Source: CAD feature listing. Evaluate the final solid. Frame: model axes, mm. A direction names the side the tool comes from. Give positions to 0.01 mm unless a question says otherwise; leave off trailing zeros. Loops run counter-clockwise (first coordinate to the right, second up) from the corner with the lowest first, then second, coordinate; pieces in that order, holes last. Notation, with made-up numbers: (29.5, -39.5) -> (63.5, -39.5) arc R18 ccw to (63.5, -16.5) -> close; hole circle Ø2 at (-15, -5.75). An arc over 180 degrees is marked (long way). Answer as a JSON object with one key per item and string values. Group by question number.
from build123d import *

# Parameters (mm, degrees)
EXTRUDE_THIN1_DEPTH    = 16.002
CUT_EXTRUDE1_START     = -15.748
CUT_EXTRUDE1_OUTLINE_R = 1.3
CUT_EXTRUDE1_DEPTH     = 15.748
BOSS_EXTRUDE2_DEPTH    = 1.68
BOSS_EXTRUDE3_START    = 1.68
BOSS_EXTRUDE3_DEPTH    = 1.68
CUT_EXTRUDE2_START     = -2.384
CUT_EXTRUDE2_DEPTH     = 2.384
CUT_EXTRUDE3_DEPTH     = 2.384
CHAMFER1_SIZE          = 1.7
CHAMFER2_SIZE          = 2.38
SKETCH10_W             = 17
SKETCH10_H             = 13.5
BOSS_EXTRUDE4_DEPTH    = 12
SKETCH11_R             = 5.6
SKETCH11_R_2           = 5
BOSS_EXTRUDE5_DEPTH    = 15
FILLET1_R              = 4


# Read off the part's stored shape, not the designer's step: Cut-Extrude1
with BuildPart() as part:
    # Sketch1 → Extrude-Thin1 (new body)
    with BuildSketch(Plane.XY):
        with BuildLine():
            Line((-42.06875, -12.7), (-35.433, -12.7))
            ThreePointArc((-35.433, -12.7), (-33.636948776, -11.956051224), (-32.893, -10.16))
            Line((-32.893, -10.16), (-32.893, -2.54))
            ThreePointArc((-32.893, -2.54), (-32.149051224, -0.743948776), (-30.353, 0))
            Line((-30.353, 0), (30.353, 0))
            ThreePointArc((30.353, 0), (32.149051224, -0.743948776), (32.893, -2.54))
            Line((32.893, -2.54), (32.893, -10.16))
            ThreePointArc((32.893, -10.16), (33.636948776, -11.956051224), (35.433, -12.7))
            Line((35.433, -12.7), (42.06875, -12.7))
            Line((42.06875, -12.7), (42.06875, -15.748))
            Line((42.06875, -15.748), (35.433, -15.748))
            ThreePointArc((35.433, -15.748), (31.481687307, -14.111312693), (29.845, -10.16))
            Line((29.845, -10.16), (29.845, -3.048))
            Line((29.845, -3.048), (-29.845, -3.048))
            Line((-29.845, -3.048), (-29.845, -10.16))
            ThreePointArc((-29.845, -10.16), (-31.481687307, -14.111312693), (-35.433, -15.748))
            Line((-35.433, -15.748), (-42.06875, -15.748))
            Line((-42.06875, -15.748), (-42.06875, -12.7))
        make_face()
    extrude(amount=-EXTRUDE_THIN1_DEPTH)

    # Cut-Extrude1 outline → Cut-Extrude1 (cut)
    with BuildSketch(Plane(origin=(0, 0, 0), x_dir=(1, 0, 0), z_dir=(0, 1, 0)).offset(CUT_EXTRUDE1_START)):
        with BuildLine():
            Line((35.433, 13.462), (-35.433, 13.462))
            ThreePointArc((-35.433, 13.462), (-37.133, 11.762), (-35.433, 10.062))
            Line((-35.433, 10.062), (-32.893, 10.062))
            Line((-32.893, 10.062), (-32.893, 8.382))
            Line((-32.893, 8.382), (-1.27, 8.382))
            Line((-1.27, 8.382), (-1.27, 12.446))
            Line((-1.27, 12.446), (32.893, 12.446))
            Line((32.893, 12.446), (32.893, 10.062))
            Line((32.893, 10.062), (35.433, 10.062))
            ThreePointArc((35.433, 10.062), (37.133, 11.762), (35.433, 13.462))
        make_face()
        with BuildLine():
            Line((32.893, 5.94), (32.893, 7.62))
            Line((32.893, 7.62), (1.27, 7.62))
            Line((1.27, 7.62), (1.27, 3.556))
            Line((1.27, 3.556), (-32.893, 3.556))
            Line((-32.893, 3.556), (-32.893, 5.94))
            Line((-32.893, 5.94), (-35.433, 5.94))
            ThreePointArc((-35.433, 5.94), (-37.133, 4.24), (-35.433, 2.54))
            Line((-35.433, 2.54), (35.433, 2.54))
            ThreePointArc((35.433, 2.54), (37.133, 4.24), (35.433, 5.94))
            Line((35.433, 5.94), (32.893, 5.94))
        make_face()
        with BuildLine():
            Line((42.06875, 16.002), (35.433, 16.002))
            ThreePointArc((35.433, 16.002), (40.193949205, 13.198335352), (42.06875, 8.001))
            Line((42.06875, 8.001), (42.06875, 16.002))
        make_face()
        with BuildLine():
            Line((42.06875, 0), (42.06875, 8.001))
            ThreePointArc((42.06875, 8.001), (40.193949205, 2.803664648), (35.433, 0))
            Line((35.433, 0), (42.06875, 0))
        make_face()
        with BuildLine():
            ThreePointArc((-42.06875, 8.001), (-40.193949205, 13.198335352), (-35.433, 16.002))
            Line((-35.433, 16.002), (-42.06875, 16.002))
            Line((-42.06875, 16.002), (-42.06875, 8.001))
        make_face()
        with BuildLine():
            ThreePointArc((-35.433, 0), (-40.193949205, 2.803664648), (-42.06875, 8.001))
            Line((-42.06875, 8.001), (-42.06875, 0))
            Line((-42.06875, 0), (-35.433, 0))
        make_face()
        with Locations((38.750875, 8.001)):
            Circle(CUT_EXTRUDE1_OUTLINE_R)
        with Locations((-38.750875, 8.001)):
            Circle(CUT_EXTRUDE1_OUTLINE_R)
    extrude(amount=CUT_EXTRUDE1_DEPTH, mode=Mode.SUBTRACT)

    # Sketch6 → Boss-Extrude2 (add)
    with BuildSketch(Plane(origin=(0, 0, -8.382), x_dir=(-1, 0, 0), z_dir=(0, 0, -1))):
        with BuildLine():
            Line((32.893, -10.16), (32.893, -6.604))
            Line((32.893, -6.604), (29.845, -6.604))
            Line((29.845, -6.604), (29.845, -10.16))
            ThreePointArc((29.845, -10.16), (30.667537588, -13.078237824), (32.893, -15.137363157))
            Line((32.893, -15.137363157), (32.893, -10.16))
        make_face()
    extrude(amount=BOSS_EXTRUDE2_DEPTH)

    # Sketch7 → Boss-Extrude3 (add)
    with BuildSketch(Plane.XY.offset(-7.62).offset(BOSS_EXTRUDE3_START)):
        with BuildLine():
            Line((32.893, -10.16), (32.893, -6.6))
            Line((32.893, -6.6), (29.845, -6.604))
            Line((29.845, -6.604), (29.845, -10.16))
            ThreePointArc((29.845, -10.16), (30.667537588, -13.078237824), (32.893, -15.137363157))
            Line((32.893, -15.137363157), (32.893, -10.16))
        make_face()
    extrude(amount=-BOSS_EXTRUDE3_DEPTH)

    # Sketch8 → Cut-Extrude2 (cut)
    with BuildSketch(Plane(origin=(0, 0, -12.446), x_dir=(-1, 0, 0), z_dir=(0, 0, -1)).offset(CUT_EXTRUDE2_START)):
        with BuildLine():
            Line((-32.893, -15.137363157), (-32.893, -6.6))
            Line((-32.893, -6.6), (-29.845, -6.604))
            Line((-29.845, -6.604), (-29.845, -10.16))
            ThreePointArc((-29.845, -10.16), (-30.667537588, -13.078237824), (-32.893, -15.137363157))
        make_face()
    extrude(amount=CUT_EXTRUDE2_DEPTH, mode=Mode.SUBTRACT)

    # Sketch9 → Cut-Extrude3 (cut)
    with BuildSketch(Plane.XY.offset(-3.556)):
        with BuildLine():
            Line((-32.893, -15.137363157), (-32.893, -6.604))
            Line((-32.893, -6.604), (-29.845, -6.604))
            Line((-29.845, -6.604), (-29.845, -10.16))
            ThreePointArc((-29.845, -10.16), (-30.667537588, -13.078237824), (-32.893, -15.137363157))
        make_face()
    extrude(amount=-CUT_EXTRUDE3_DEPTH, mode=Mode.SUBTRACT)

    # Chamfer1
    # the kernel refuses this chamfer: 1.7 mm, written as the material it adds along each edge
    # the kernel refuses this chamfer: 1.7 mm, written as the material it takes off along each edge
    with BuildSketch(Plane(origin=(-37.26486108, -6.604, -10.062), x_dir=(0, -0.9996219169112968, -0.02749587661058687), z_dir=(1, 0, 0))) as chamfer1_2_piece_1_section:
        Polygon((CHAMFER1_SIZE * 0.999621916911, -CHAMFER1_SIZE * 0.0274958766106), (-CHAMFER1_SIZE * 0.0274958766106, -CHAMFER1_SIZE * 0.999621916911), (0, 0), align=None)
    chamfer1_2_piece_1 = extrude(amount=11.791722159, mode=Mode.PRIVATE)
    chamfer1_2_piece_1 = split(chamfer1_2_piece_1, bisect_by=Plane(origin=(-31.369, -7.170744186, -8.382), z_dir=(0, 0, -1)), keep=Keep.TOP, mode=Mode.PRIVATE)
    add(chamfer1_2_piece_1, mode=Mode.SUBTRACT)
    with BuildSketch(Plane(origin=(37.264857315, -6.594262654, -5.94), x_dir=(0.00131183865632537, -0.9996210561251475, 0.02749587661058631), z_dir=(-0.999999138888279, -0.0013123348279305267, 0))) as chamfer1_2_piece_2_section:
        Polygon((CHAMFER1_SIZE * 0.999621916911, -CHAMFER1_SIZE * 0.0274958766106), (-CHAMFER1_SIZE * 0.0274958766106, -CHAMFER1_SIZE * 0.999621916911), (0, 0), align=None)
    chamfer1_2_piece_2 = extrude(amount=11.791724784, mode=Mode.PRIVATE)
    chamfer1_2_piece_2 = split(chamfer1_2_piece_2, bisect_by=Plane(origin=(31.369, -7.168744674, -7.62), z_dir=(0, 0, 1)), keep=Keep.TOP, mode=Mode.PRIVATE)
    add(chamfer1_2_piece_2, mode=Mode.SUBTRACT)

    # Chamfer2
    chamfer2_edges = [part.edges().sort_by_distance(p)[0] for p in [
        (31.369, -6.602, -10.062),
        (-31.369, -6.604, -5.94),
    ]]
    chamfer(chamfer2_edges, length=CHAMFER2_SIZE)

    # Sketch10 → Boss-Extrude4 (add)
    with BuildSketch(Plane.XZ.offset(3.048)):
        with Locations((-21.345, -8.001)):
            Rectangle(SKETCH10_W, SKETCH10_H)
    extrude(amount=BOSS_EXTRUDE4_DEPTH)

    # Sketch11 → Boss-Extrude5 (add)
    with BuildSketch(Plane(origin=(-12.845, 0, 0), x_dir=(0, 0, -1), z_dir=(1, 0, 0))):
        with Locations(Location((8.001, -9.048, 0), (0, 0, 270))):
            Circle(SKETCH11_R)
        with Locations(Location((8.001, -9.048, 0), (0, 0, 90))):
            Circle(SKETCH11_R_2, mode=Mode.SUBTRACT)
    extrude(amount=BOSS_EXTRUDE5_DEPTH)

    # Fillet1
    fillet1_edges = [part.edges().sort_by_distance(p)[0] for p in [
        (-21.345, -15.048, -14.751),
        (-21.345, -15.048, -1.251),
    ]]
    fillet(fillet1_edges, radius=FILLET1_R)


solid = part.part
(1) Mould query, pull axis Z, two halves, no side actions, for faces 5 (the face through (1.27, -2, -6)), 6 (the face through (32.893, -6, -15)), 7 (the face through (-5.45, -14.221, -5.856)). Classes: pulls with the +Z half, pulls with the -Z half, needs draft (parallel to the pull), parting line crosses it, or undercut.
(2) Section query D-D on x = -19.5. Return the cut outline in (y, z).
(3) Material intervals for line 1 (Z direction, x = -8, y = -2.25); line 2 (X direction, y = -7.75, z = -9.75) (3 decimals); line 3 (Y direction, x = -9, z = -4.25), sorted ascending. Write a range as from..to.
(4) Section query C-C on x = 6. Return the cut outline in (y, z), plus the area to 3 significant figures.
(5) Section query A-A on x = -2.5. Return the cut outline in (y, z), plus the area to 3 significant figures.
(6) First-contact query: pin 1 (8 mm diameter, centred on y = -8, z = -6, fed in from +X); pin 2 (1 mm diameter, centred on x = -32.5, y = -4, fed in from +Z); pin 3 (5 mm diameter, centred on x = 22, z = -2, fed in from -Y); pin 4 (3.5 mm diameter, centred on y = -8, z = -10.5, fed in from +X). Flat tips, straight axial feed; report the tip coordinate or a pass-through.
(7) Access query for faces 1 (the face through (31.525, -14.155, -14.714)), 2 (the face through (32.893, -6, -9)), 3 (the face through (-32.893, -6, -7)), 4 (the face through (0.5, -2.7, -13.462)). Directions: +Z, -Z, +X, -X, +Y, -Y. A direction counts if a zero-diameter tool reaches every point of the face in a straight line with its end or side. Return the directions, or none.
(8) Section query B-B on y = -1.25. Return the cut outline in (x, z).
Result:
{
 "1": {"face 5": "undercut", "face 6": "needs draft", "face 7": "parting line crosses it"},
 "2": {"outline": "(-15.05, -10.75) arc R4 ccw to (-11.05, -14.75) -> (-3.05, -14.75) -> (-3.05, -16) -> (0, -16) -> (0, -13.46) -> (-3.05, -13.46) -> (-3.05, -8.38) -> (0, -8.38) -> (0, -3.56) -> (-3.05, -3.56) -> (-3.05, -2.54) -> (0, -2.54) -> (0, 0) -> (-3.05, 0) -> (-3.05, -1.25) -> (-11.05, -1.25) arc R4 ccw to (-15.05, -5.25) -> close"},
 "3": {"line 1": "-16..-13.46, -8.38..-3.56, -2.54..0", "line 2": "-29.845..-12.845, 29.845..32.893", "line 3": "-13.21..-12.35, -5.74..-4.89, -3.05..0"},
 "4": {"outline": "(-3.05, -16) -> (0, -16) -> (0, -13.46) -> (-3.05, -13.46) -> close; (-3.05, -12.45) -> (0, -12.45) -> (0, -7.62) -> (-3.05, -7.62) -> close; (-3.05, -2.54) -> (0, -2.54) -> (0, 0) -> (-3.05, 0) -> close", "area": "30.2 mm²"},
 "5": {"outline": "circle Ø11.2 at (-9.05, -8); (-3.05, -16) -> (0, -16) -> (0, -13.46) -> (-3.05, -13.46) -> close; (-3.05, -8.38) -> (0, -8.38) -> (0, -3.56) -> (-3.05, -3.56) -> close; (-3.05, -2.54) -> (0, -2.54) -> (0, 0) -> (-3.05, 0) -> close; hole circle Ø10 at (-9.05, -8)", "area": "50.2 mm²"},
 "6": {"pin 1": "x = 33.68", "pin 2": "z = 0", "pin 3": "y = -3.05", "pin 4": "x = 32.89"},
 "7": {"face 1": "+Z, -Z, -Y", "face 2": "+Z, -Z, +X, +Y", "face 3": "+Z, -Z, -X, +Y", "face 4": "+Y"},
 "8": {"outline": "(-32.54, -16) -> (32.54, -16) -> (32.54, -13.46) -> (-32.54, -13.46) -> close; (-32.54, -8.38) -> (-1.27, -8.38) -> (-1.27, -12.45) -> (32.54, -12.45) -> (32.54, -7.62) -> (1.27, -7.62) -> (1.27, -3.56) -> (-32.54, -3.56) -> close; (-32.54, -2.54) -> (32.54, -2.54) -> (32.54, 0) -> (-32.54, 0) -> close"}
}
